```python
from build123d import *

# Parameters (mm, degrees)
SKETCH1_R           = 4.5
BOSS_EXTRUDE1_DEPTH = 6
SKETCH2_R           = 6
SKETCH2_R_2         = 3.5
BOSS_EXTRUDE2_DEPTH = 11
BOSS_EXTRUDE3_START = -6
SKETCH3_R           = 3.5
SKETCH3_R_2         = 1.65
BOSS_EXTRUDE3_DEPTH = 7
BOSS_EXTRUDE4_DEPTH = 5


with BuildPart() as part:
    # Sketch1 → Boss-Extrude1 (new body)
    with BuildSketch(Plane.XY):
        with BuildLine():
            Line((102.949952293, 87.641492111), (84.646703629, 84.03494065))
            ThreePointArc((84.646703629, 84.03494065), (80.592912741, 81.612614555), (78.999992436, 77.166999954))
            Line((78.999992436, 77.166999954), (78.999992436, -2.166999954))
            ThreePointArc((78.999992436, -2.166999954), (80.592912741, -6.612614555), (84.646703629, -9.03494065))
            Line((84.646703629, -9.03494065), (102.949952293, -12.641492111))
            ThreePointArc((102.949952293, -12.641492111), (107.293299673, -15.2368415), (109, -20))
            Line((109, -20), (109, -25))
            ThreePointArc((109, -25), (103.458898596, -32.239662719), (95.023275656, -28.781804036))
            ThreePointArc((95.023275656, -28.781804036), (93.036589613, -26.607931656), (90.331621742, -25.443547107))
            Line((90.331621742, -25.443547107), (-1.449952293, -7.358507889))
            ThreePointArc((-1.449952293, -7.358507889), (-7.358507889, 1.449952293), (1.449952293, 7.358507889))
            Line((1.449952293, 7.358507889), (55.646703629, -3.320654936))
            ThreePointArc((55.646703629, -3.320654936), (61.445607037, -1.859793935), (63.999992436, 3.54728576))
            Line((63.999992436, 3.54728576), (63.999992436, 71.45271424))
            ThreePointArc((63.999992436, 71.45271424), (61.445607037, 76.859793935), (55.646703629, 78.320654936))
            Line((55.646703629, 78.320654936), (1.449952293, 67.641492111))
            ThreePointArc((1.449952293, 67.641492111), (-7.358507889, 73.550047707), (-1.449952293, 82.358507889))
            Line((-1.449952293, 82.358507889), (90.331621742, 100.443547107))
            ThreePointArc((90.331621742, 100.443547107), (93.036589613, 101.607931655), (95.023275656, 103.781804036))
            ThreePointArc((95.023275656, 103.781804036), (103.458898596, 107.239662719), (109, 100))
            Line((109, 100), (109, 95))
            ThreePointArc((109, 95), (107.293299673, 90.2368415), (102.949952293, 87.641492111))
        make_face()
        Circle(SKETCH1_R, mode=Mode.SUBTRACT)
        with Locations(Location((0, 75, 0), (0, 0, 180))):
            Circle(SKETCH1_R, mode=Mode.SUBTRACT)
        with BuildLine():
            Line((102.6, -25), (102.6, -20))
            ThreePointArc((102.6, -20), (101.5, -18.9), (100.4, -20))
            Line((100.4, -20), (100.4, -25))
            ThreePointArc((100.4, -25), (101.5, -26.1), (102.6, -25))
        make_face(mode=Mode.SUBTRACT)
        with BuildLine():
            Line((100.4, 100), (100.4, 95))
            ThreePointArc((100.4, 95), (101.5, 93.9), (102.6, 95))
            Line((102.6, 95), (102.6, 100))
            ThreePointArc((102.6, 100), (101.5, 101.1), (100.4, 100))
        make_face(mode=Mode.SUBTRACT)
    extrude(amount=BOSS_EXTRUDE1_DEPTH)

    # Sketch2 → Boss-Extrude2 (add)
    # profile 1 of 2: a face of its own
    with BuildSketch(Plane.XY.offset(6)):
        with Locations((0, 75)):
            Circle(SKETCH2_R)
        with Locations((0, 75)):
            Circle(SKETCH2_R_2, mode=Mode.SUBTRACT)
    # profile 2 of 2: a face of its own
    with BuildSketch(Plane.XY.offset(6)):
        Circle(SKETCH2_R)
        Circle(SKETCH2_R_2, mode=Mode.SUBTRACT)
    extrude(amount=BOSS_EXTRUDE2_DEPTH)

    # Sketch3 → Boss-Extrude3 (add)
    # profile 1 of 2: a face of its own
    with BuildSketch(Plane(origin=(0, 0, 0), x_dir=(-1, 0, 0), z_dir=(0, 0, -1)).offset(BOSS_EXTRUDE3_START)):
        with Locations(Location((0, 75, 0), (0, 0, 180))):
            Circle(SKETCH3_R)
        with Locations((0, 75)):
            Circle(SKETCH3_R_2, mode=Mode.SUBTRACT)
    # profile 2 of 2: a face of its own
    with BuildSketch(Plane(origin=(0, 0, 0), x_dir=(-1, 0, 0), z_dir=(0, 0, -1)).offset(BOSS_EXTRUDE3_START)):
        with Locations(Location((0, 0, 0), (0, 0, 180))):
            Circle(SKETCH3_R)
        Circle(SKETCH3_R_2, mode=Mode.SUBTRACT)
    extrude(amount=-BOSS_EXTRUDE3_DEPTH)

    # Sketch4 → Boss-Extrude4 (add)
    # profile 1 of 2: a face of its own
    with BuildSketch(Plane.XY.offset(6)):
        with BuildLine():
            Line((94, -20), (94, -25))
            ThreePointArc((94, -25), (101.5, -32.5), (109, -25))
            Line((109, -25), (109, -20))
            ThreePointArc((109, -20), (101.5, -12.5), (94, -20))
        make_face()
        Polygon((101.5, -15.843078062), (97.9, -17.921539031), (97.9, -27.078460969), (101.5, -29.156921938), (105.1, -27.078460969), (105.1, -17.921539031), align=None, mode=Mode.SUBTRACT)
    # profile 2 of 2: a face of its own
    with BuildSketch(Plane.XY.offset(6)):
        with BuildLine():
            Line((94, 100), (94, 95))
            ThreePointArc((94, 95), (101.5, 87.5), (109, 95))
            Line((109, 95), (109, 100))
            ThreePointArc((109, 100), (101.5, 107.5), (94, 100))
        make_face()
        Polygon((101.5, 104.156921938), (97.9, 102.078460969), (97.9, 92.921539031), (101.5, 90.843078062), (105.1, 92.921539031), (105.1, 102.078460969), align=None, mode=Mode.SUBTRACT)
    extrude(amount=BOSS_EXTRUDE4_DEPTH)


solid = part.part
```
Check sheet for the modelled part. Datum: model origin and axes. Units: mm. A direction names the side the tool comes from. Round coordinates to 2 decimals unless told otherwise and drop trailing zeros. Order: outer loops, then holes, each group sorted by start corner. A loop starts at its lowest first (then second) coordinate and runs counter-clockwise, first axis right, second up.
1) Scan lines: line 1 (Y direction, x = 0, z = 14.3); line 2 (Y direction, x = 0, z = 7.75); line 3 (Z direction, x = 69.5, y = -2.5). Record each from-to range of solid material in increasing order.
2) Go/stop test with flat-tipped pins: pin 1 Ø12 at (x, y) = (38, 6.5) entering from +Z; pin 2 Ø1.5 at (y, z) = (70, 12) entering from -X; pin 3 Ø2 at (x, y) = (-1, 1.5) entering from +Z; pin 4 Ø7.5 at (x, y) = (103.5, -22.5) entering from +Z. Record where each tip stops, or that it passes through.
3) Mould release check, pull along Y, two halves, no side actions. Record for faces 1 (the flat face through (3, 72, 17)), 2 (the flat face through (103, -22, 6)), 3 (the flat face through (103, 98, 6)), 4 (the cylindrical face through (93, 101.58, 2.96)): +Y half, -Y half, draft (parallel to the pull), parting line (faces both ways), or undercut.
4) Section check C-C (x = 92.5). Record the boundary of the cut face in (y, z).
5) Section check B-B (y = 0). Record the boundary of the cut face in (x, z), and give its area (3 significant figures).
6) Section check A-A (z = 14.5). Record the boundary of the cut face in (x, y).
7) Section check D-D (y = 19). Record the boundary of the cut face in (x, z).
8) Tool access check on faces 5 (the cylindrical face through (-6, 0, 11)), 6 (the flat face through (43.798, 91.274, 2.958)), 7 (the cylindrical face through (0.59, 70.54, 2.96)), 8 (the cylindrical face through (93.07, -26.63, 2.96)), 9 (the cylindrical face through (80.55, -6.56, 2.96)). Record the directions out of +Z, -Z, +X, -X, +Y, -Y that give a thin tool (end or side, any length) a straight path to the whole face; none if there is none.
Result:
1. line 1: y = -6 to -3.5, 3.5 to 6, 69 to 71.5, 78.5 to 81
1. line 2: y = -6 to -1.65, 1.65 to 6, 69 to 73.35, 76.65 to 81
1. line 3: z = 0 to 6
2. pin 1: passes through
2. pin 2: stops at x = -4.24
2. pin 3: stops at z = 13
2. pin 4: stops at z = 11
3. face 1: draft
3. face 2: undercut
3. face 3: undercut
3. face 4: +Y half
4. outline: (-26.26, 0) - (-10.58, 0) - (-10.58, 6) - (-26.26, 6) - close; (85.58, 0) - (101.26, 0) - (101.26, 6) - (85.58, 6) - close
5. outline: (-7.5, 0) - (-4.5, 0) - (-4.5, 6) - (-1.65, 6) - (-1.65, 13) - (-3.5, 13) - (-3.5, 17) - (-6, 17) - (-6, 6) - (-7.5, 6) - close; (1.65, 6) - (4.5, 6) - (4.5, 0) - (38.79, 0) - (38.79, 6) - (6, 6) - (6, 17) - (3.5, 17) - (3.5, 13) - (1.65, 13) - close; (63.03, 0) - (79, 0) - (79, 6) - (63.03, 6) - close
5. area: 400 mm2
6. outline: circle Ø12 at (0, 0); circle Ø12 at (0, 75); hole circle Ø7 at (0, 0); hole circle Ø7 at (0, 75)
7. outline: (64, 0) - (79, 0) - (79, 6) - (64, 6) - close
8. face 5: +Z
8. face 6: +Z, -Z, -X, +Y
8. face 7: -Z
8. face 8: +Z, -Z, -X, -Y
8. face 9: +Z, -Z, +X
